Model file for the job. Use its own axes, mm. Face numbers are marked on the shaded views. A direction names the side the tool comes from. Coordinates: 2 decimals unless noted, no trailing zeros. Write each loop counter-clockwise with the first axis right and the second up, starting at its lowest first coordinate (ties: lowest second). Pieces come first, ordered by that corner, then holes.
Q1. Band-saw the part on B-B, the plane y = 74. Write the cut outline in (x, z), plus the area to 3 significant figures.
Q2. Pull direction X, two halves, no side cores. Call the marked faces 1, 2 and 3: released by +X, released by -X, zero draft, split by the parting line, or undercut.
Q3. Drill centre lines: probe 1 along X at (y, z) = (51.5, -21); probe 2 along Y at (x, z) = (24, -14); probe 3 along Z at (x, y) = (-20.75, 70.5). Where is each one in solid material? Low to high.
Q4. Pin check, flat tips, straight feed: P1, Ø5, axis at x = 22.5, y = 16.75, coming from the +Z side; P2, Ø9, axis at x = -22.5, y = 16.75, coming from the -Z side; P3, Ø1.3, axis at x = 25, y = 53, coming from the +Z side; P4, Ø3, axis at x = 15, z = -21, coming from the -Y side. Stop position of each tip, or through.
Q5. Band-saw the part on C-C, the plane z = -52. Write the cut outline in (x, y).
Q6. Band-saw the part on A-A, the plane x = 15.5. Write the cut outline in (y, z).
Q7. Band-saw the part on D-D, the plane x = 1. Write the cut outline in (y, z).
Q8. Which spindle directions (+Z, -Z, +X, -X, +Y, -Y) get a long thin tool onto all of the face, cutting with end or side? Do the marked faces 4 and 5. Say none if no direction does.
from build123d import *

# Parameters (mm, degrees)
SKETCH2_W           = 5
SKETCH2_H           = 50
BOSS_EXTRUDE1_DEPTH = 30
CUT_EXTRUDE1_REACH  = 66.607
SKETCH3_R           = 2.25
SKETCH6_W           = 47
SKETCH6_H           = 34
BOSS_EXTRUDE3_DEPTH = 60
SKETCH7_R           = 4
CUT_EXTRUDE2_DEPTH  = 2.3
CUT_EXTRUDE3_REACH  = 77.168
SKETCH8_R           = 11.5
SKETCH8_R_2         = 4.15
SKETCH8_R_3         = 1.75
CHAMFER1_SIZE       = 13
SKETCH9_R           = 3
CUT_EXTRUDE4_DEPTH  = 17
CHAMFER2_SIZE       = 9
SKETCH3_2_R         = 2.25
CUT_EXTRUDE5_DEPTH  = 5


with BuildPart() as part:
    # Sketch2 → Boss-Extrude1 (new, symmetric)
    with BuildSketch(Plane(origin=(0, 0, 0), x_dir=(0, 0, -1), z_dir=(1, 0, 0))):
        with Locations((13, 32)):
            Rectangle(SKETCH2_W, SKETCH2_H)
    extrude(amount=BOSS_EXTRUDE1_DEPTH, both=True)

    # Sketch3 → Cut-Extrude1 (cut, up to next)
    with BuildSketch(Plane.XY.offset(-10.5), mode=Mode.PRIVATE) as cut_extrude1_sk1:
        with Locations((-22.5, 16.75)):
            Circle(SKETCH3_R)
    cut_extrude1_tool1 = extrude(cut_extrude1_sk1.sketch, amount=-CUT_EXTRUDE1_REACH, mode=Mode.PRIVATE) & part.part
    # Sketch3 → Cut-Extrude1 (cut, up to next)
    with BuildSketch(Plane.XY.offset(-10.5), mode=Mode.PRIVATE) as cut_extrude1_sk2:
        with Locations((-7.5, 16.75)):
            Circle(SKETCH3_R)
    cut_extrude1_tool2 = extrude(cut_extrude1_sk2.sketch, amount=-CUT_EXTRUDE1_REACH, mode=Mode.PRIVATE) & part.part
    # Sketch3 → Cut-Extrude1 (cut, up to next)
    with BuildSketch(Plane.XY.offset(-10.5), mode=Mode.PRIVATE) as cut_extrude1_sk3:
        with Locations((7.5, 16.75)):
            Circle(SKETCH3_R)
    cut_extrude1_tool3 = extrude(cut_extrude1_sk3.sketch, amount=-CUT_EXTRUDE1_REACH, mode=Mode.PRIVATE) & part.part
    # Sketch3 → Cut-Extrude1 (cut, up to next)
    with BuildSketch(Plane.XY.offset(-10.5), mode=Mode.PRIVATE) as cut_extrude1_sk4:
        with Locations((22.5, 16.75)):
            Circle(SKETCH3_R)
    cut_extrude1_tool4 = extrude(cut_extrude1_sk4.sketch, amount=-CUT_EXTRUDE1_REACH, mode=Mode.PRIVATE) & part.part
    # Sketch3 → Cut-Extrude1 (cut, up to next)
    with BuildSketch(Plane.XY.offset(-10.5), mode=Mode.PRIVATE) as cut_extrude1_sk5:
        with Locations((-24, 52)):
            Circle(SKETCH3_R)
    cut_extrude1_tool5 = extrude(cut_extrude1_sk5.sketch, amount=-CUT_EXTRUDE1_REACH, mode=Mode.PRIVATE) & part.part
    # Sketch3 → Cut-Extrude1 (cut, up to next)
    with BuildSketch(Plane.XY.offset(-10.5), mode=Mode.PRIVATE) as cut_extrude1_sk6:
        with Locations((-6, 52)):
            Circle(SKETCH3_R)
    cut_extrude1_tool6 = extrude(cut_extrude1_sk6.sketch, amount=-CUT_EXTRUDE1_REACH, mode=Mode.PRIVATE) & part.part
    # Sketch3 → Cut-Extrude1 (cut, up to next)
    with BuildSketch(Plane.XY.offset(-10.5), mode=Mode.PRIVATE) as cut_extrude1_sk7:
        with Locations((-24, 28)):
            Circle(SKETCH3_R)
    cut_extrude1_tool7 = extrude(cut_extrude1_sk7.sketch, amount=-CUT_EXTRUDE1_REACH, mode=Mode.PRIVATE) & part.part
    # Sketch3 → Cut-Extrude1 (cut, up to next)
    with BuildSketch(Plane.XY.offset(-10.5), mode=Mode.PRIVATE) as cut_extrude1_sk8:
        with Locations((-6, 28)):
            Circle(SKETCH3_R)
    cut_extrude1_tool8 = extrude(cut_extrude1_sk8.sketch, amount=-CUT_EXTRUDE1_REACH, mode=Mode.PRIVATE) & part.part
    # Sketch3 → Cut-Extrude1 (cut, up to next)
    with BuildSketch(Plane.XY.offset(-10.5), mode=Mode.PRIVATE) as cut_extrude1_sk9:
        with Locations(Location((6, 28, 0), (0, 0, 90))):
            Circle(SKETCH3_R)
    cut_extrude1_tool9 = extrude(cut_extrude1_sk9.sketch, amount=-CUT_EXTRUDE1_REACH, mode=Mode.PRIVATE) & part.part
    # Sketch3 → Cut-Extrude1 (cut, up to next)
    with BuildSketch(Plane.XY.offset(-10.5), mode=Mode.PRIVATE) as cut_extrude1_sk10:
        with Locations(Location((24, 28, 0), (0, 0, 90))):
            Circle(SKETCH3_R)
    cut_extrude1_tool10 = extrude(cut_extrude1_sk10.sketch, amount=-CUT_EXTRUDE1_REACH, mode=Mode.PRIVATE) & part.part
    # Sketch3 → Cut-Extrude1 (cut, up to next)
    with BuildSketch(Plane.XY.offset(-10.5), mode=Mode.PRIVATE) as cut_extrude1_sk11:
        with Locations(Location((6, 52, 0), (0, 0, 90))):
            Circle(SKETCH3_R)
    cut_extrude1_tool11 = extrude(cut_extrude1_sk11.sketch, amount=-CUT_EXTRUDE1_REACH, mode=Mode.PRIVATE) & part.part
    # Sketch3 → Cut-Extrude1 (cut, up to next)
    with BuildSketch(Plane.XY.offset(-10.5), mode=Mode.PRIVATE) as cut_extrude1_sk12:
        with Locations(Location((24, 52, 0), (0, 0, 90))):
            Circle(SKETCH3_R)
    cut_extrude1_tool12 = extrude(cut_extrude1_sk12.sketch, amount=-CUT_EXTRUDE1_REACH, mode=Mode.PRIVATE) & part.part
    add(cut_extrude1_tool1.solids().sort_by_distance((-22.5, 16.75, -10.5))[0], mode=Mode.SUBTRACT)
    add(cut_extrude1_tool2.solids().sort_by_distance((-7.5, 16.75, -10.5))[0], mode=Mode.SUBTRACT)
    add(cut_extrude1_tool3.solids().sort_by_distance((7.5, 16.75, -10.5))[0], mode=Mode.SUBTRACT)
    add(cut_extrude1_tool4.solids().sort_by_distance((22.5, 16.75, -10.5))[0], mode=Mode.SUBTRACT)
    add(cut_extrude1_tool5.solids().sort_by_distance((-24, 52, -10.5))[0], mode=Mode.SUBTRACT)
    add(cut_extrude1_tool6.solids().sort_by_distance((-6, 52, -10.5))[0], mode=Mode.SUBTRACT)
    add(cut_extrude1_tool7.solids().sort_by_distance((-24, 28, -10.5))[0], mode=Mode.SUBTRACT)
    add(cut_extrude1_tool8.solids().sort_by_distance((-6, 28, -10.5))[0], mode=Mode.SUBTRACT)
    add(cut_extrude1_tool9.solids().sort_by_distance((6, 28, -10.5))[0], mode=Mode.SUBTRACT)
    add(cut_extrude1_tool10.solids().sort_by_distance((24, 28, -10.5))[0], mode=Mode.SUBTRACT)
    add(cut_extrude1_tool11.solids().sort_by_distance((6, 52, -10.5))[0], mode=Mode.SUBTRACT)
    add(cut_extrude1_tool12.solids().sort_by_distance((24, 52, -10.5))[0], mode=Mode.SUBTRACT)

    # Sketch6 → Boss-Extrude3 (add)
    with BuildSketch(Plane(origin=(30, 0, 0), x_dir=(0, 0, -1), z_dir=(1, 0, 0))):
        with Locations((34, 62)):
            Rectangle(SKETCH6_W, SKETCH6_H)
    extrude(amount=-BOSS_EXTRUDE3_DEPTH)

    # Sketch7 → Cut-Extrude2 (cut)
    with BuildSketch(Plane(origin=(0, 0, -15.5), x_dir=(-1, 0, 0), z_dir=(0, 0, -1))):
        with Locations(Location((22.5, 16.75, 0), (0, 0, 90))):
            Circle(SKETCH7_R)
        with Locations(Location((24, 28, 0), (0, 0, 90))):
            Circle(SKETCH7_R)
        with Locations(Location((7.5, 16.75, 0), (0, 0, 90))):
            Circle(SKETCH7_R)
        with Locations(Location((-7.5, 16.75, 0), (0, 0, 90))):
            Circle(SKETCH7_R)
        with Locations(Location((-22.5, 16.75, 0), (0, 0, 90))):
            Circle(SKETCH7_R)
        with Locations(Location((6, 28, 0), (0, 0, 90))):
            Circle(SKETCH7_R)
        with Locations(Location((-6, 28, 0), (0, 0, 270))):
            Circle(SKETCH7_R)
        with Locations(Location((-24, 28, 0), (0, 0, 270))):
            Circle(SKETCH7_R)
    extrude(amount=-CUT_EXTRUDE2_DEPTH, mode=Mode.SUBTRACT)

    # Sketch8 → Cut-Extrude3 (cut, up to next)
    with BuildSketch(Plane.XZ.offset(-45), mode=Mode.PRIVATE) as cut_extrude3_sk1:
        with Locations(Location((0, -36.5, 0), (0, 0, 270))):
            Circle(SKETCH8_R)
    cut_extrude3_tool1 = extrude(cut_extrude3_sk1.sketch, amount=-CUT_EXTRUDE3_REACH, mode=Mode.PRIVATE) & part.part
    # Sketch8 → Cut-Extrude3 (cut, up to next)
    with BuildSketch(Plane.XZ.offset(-45), mode=Mode.PRIVATE) as cut_extrude3_sk2:
        with Locations(Location((-20.75, -36.5, 0), (0, 0, 270))):
            Circle(SKETCH8_R_2)
    cut_extrude3_tool2 = extrude(cut_extrude3_sk2.sketch, amount=-CUT_EXTRUDE3_REACH, mode=Mode.PRIVATE) & part.part
    # Sketch8 → Cut-Extrude3 (cut, up to next)
    with BuildSketch(Plane.XZ.offset(-45), mode=Mode.PRIVATE) as cut_extrude3_sk3:
        with Locations(Location((20.75, -36.5, 0), (0, 0, 90))):
            Circle(SKETCH8_R_2)
    cut_extrude3_tool3 = extrude(cut_extrude3_sk3.sketch, amount=-CUT_EXTRUDE3_REACH, mode=Mode.PRIVATE) & part.part
    # Sketch8 → Cut-Extrude3 (cut, up to next)
    with BuildSketch(Plane.XZ.offset(-45), mode=Mode.PRIVATE) as cut_extrude3_sk4:
        with Locations(Location((-15.5, -52, 0), (0, 0, 270))):
            Circle(SKETCH8_R_3)
    cut_extrude3_tool4 = extrude(cut_extrude3_sk4.sketch, amount=-CUT_EXTRUDE3_REACH, mode=Mode.PRIVATE) & part.part
    # Sketch8 → Cut-Extrude3 (cut, up to next)
    with BuildSketch(Plane.XZ.offset(-45), mode=Mode.PRIVATE) as cut_extrude3_sk5:
        with Locations(Location((15.5, -52, 0), (0, 0, 90))):
            Circle(SKETCH8_R_3)
    cut_extrude3_tool5 = extrude(cut_extrude3_sk5.sketch, amount=-CUT_EXTRUDE3_REACH, mode=Mode.PRIVATE) & part.part
    # Sketch8 → Cut-Extrude3 (cut, up to next)
    with BuildSketch(Plane.XZ.offset(-45), mode=Mode.PRIVATE) as cut_extrude3_sk6:
        with Locations(Location((15.5, -21, 0), (0, 0, 270))):
            Circle(SKETCH8_R_3)
    cut_extrude3_tool6 = extrude(cut_extrude3_sk6.sketch, amount=-CUT_EXTRUDE3_REACH, mode=Mode.PRIVATE) & part.part
    # Sketch8 → Cut-Extrude3 (cut, up to next)
    with BuildSketch(Plane.XZ.offset(-45), mode=Mode.PRIVATE) as cut_extrude3_sk7:
        with Locations(Location((-15.5, -21, 0), (0, 0, 90))):
            Circle(SKETCH8_R_3)
    cut_extrude3_tool7 = extrude(cut_extrude3_sk7.sketch, amount=-CUT_EXTRUDE3_REACH, mode=Mode.PRIVATE) & part.part
    add(cut_extrude3_tool1.solids().sort_by_distance((0, 45, -36.5))[0], mode=Mode.SUBTRACT)
    add(cut_extrude3_tool2.solids().sort_by_distance((-20.75, 45, -36.5))[0], mode=Mode.SUBTRACT)
    add(cut_extrude3_tool3.solids().sort_by_distance((20.75, 45, -36.5))[0], mode=Mode.SUBTRACT)
    add(cut_extrude3_tool4.solids().sort_by_distance((-15.5, 45, -52))[0], mode=Mode.SUBTRACT)
    add(cut_extrude3_tool5.solids().sort_by_distance((15.5, 45, -52))[0], mode=Mode.SUBTRACT)
    add(cut_extrude3_tool6.solids().sort_by_distance((15.5, 45, -21))[0], mode=Mode.SUBTRACT)
    add(cut_extrude3_tool7.solids().sort_by_distance((-15.5, 45, -21))[0], mode=Mode.SUBTRACT)

    # Chamfer1
    chamfer1_edges = [part.edges().sort_by_distance(p)[0] for p in [
        (30, 62, -57.5),
        (-30, 62, -57.5),
    ]]
    chamfer(chamfer1_edges, length=CHAMFER1_SIZE)

    # Sketch9 → Cut-Extrude4 (cut)
    with BuildSketch(Plane.XZ.offset(-45)):
        with Locations(Location((-15.5, -21, 0), (0, 0, 270))):
            Circle(SKETCH9_R)
        with Locations(Location((-15.5, -52, 0), (0, 0, 270))):
            Circle(SKETCH9_R)
        with Locations(Location((15.5, -52, 0), (0, 0, 90))):
            Circle(SKETCH9_R)
        with Locations(Location((15.5, -21, 0), (0, 0, 90))):
            Circle(SKETCH9_R)
    extrude(amount=-CUT_EXTRUDE4_DEPTH, mode=Mode.SUBTRACT)

    # Chamfer2
    # the kernel refuses this chamfer: 9 mm, written as the material it takes off along each edge
    with BuildSketch(Plane(origin=(30, 79, -67.645146892), x_dir=(-0.9996219169112966, 0.027495876610586775, 0), z_dir=(0, 0, 1)), Plane(origin=(-30, 79, -67.645146892), x_dir=(-0.027495876610586386, -0.9996219169112969, 0), z_dir=(0, 0, 1))) as chamfer2_piece_1:
        Polygon((CHAMFER2_SIZE * 0.999621916911, CHAMFER2_SIZE * 0.0274958766106), (-CHAMFER2_SIZE * 0.0274958766106, CHAMFER2_SIZE * 0.999621916911), (0, 0), align=None)
    extrude(amount=80.290293783, mode=Mode.SUBTRACT)

    # Sketch3<2> → Cut-Extrude5 (cut)
    with BuildSketch(Plane.XY.offset(-10.5)):
        with Locations((-22.5, 16.75)):
            Circle(SKETCH3_2_R)
        with Locations((-7.5, 16.75)):
            Circle(SKETCH3_2_R)
        with Locations((7.5, 16.75)):
            Circle(SKETCH3_2_R)
        with Locations((22.5, 16.75)):
            Circle(SKETCH3_2_R)
        with Locations((-24, 52)):
            Circle(SKETCH3_2_R)
        with Locations((-6, 52)):
            Circle(SKETCH3_2_R)
        with Locations((-24, 28)):
            Circle(SKETCH3_2_R)
        with Locations((-6, 28)):
            Circle(SKETCH3_2_R)
        with Locations(Location((6, 28, 0), (0, 0, 270))):
            Circle(SKETCH3_2_R)
        with Locations(Location((24, 28, 0), (0, 0, 270))):
            Circle(SKETCH3_2_R)
        with Locations(Location((6, 52, 0), (0, 0, 90))):
            Circle(SKETCH3_2_R)
        with Locations(Location((24, 52, 0), (0, 0, 90))):
            Circle(SKETCH3_2_R)
    extrude(amount=-CUT_EXTRUDE5_DEPTH, mode=Mode.SUBTRACT)


solid = part.part
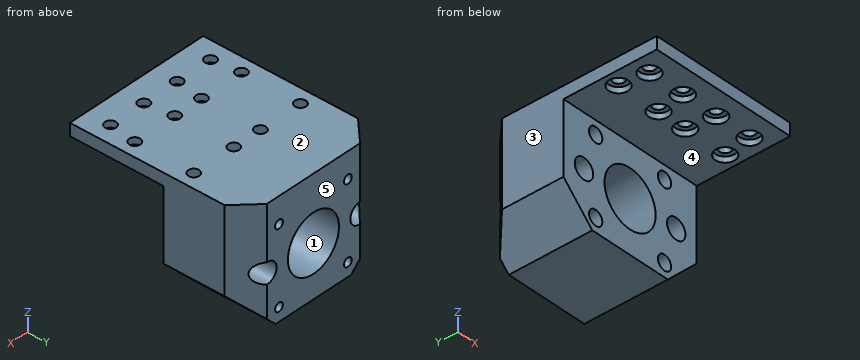
Answer sheet:
1. outline: (-26, -48.5) - (-17, -57.5) - (17, -57.5) - (26, -48.5) - (26, -10.5) - (-26, -10.5) - close; hole circle Ø8.3 at (-20.75, -36.5); hole circle Ø3.5 at (-15.5, -52); hole circle Ø3.5 at (-15.5, -21); hole circle Ø23 at (0, -36.5); hole circle Ø3.5 at (15.5, -52); hole circle Ø3.5 at (15.5, -21); hole circle Ø8.3 at (20.75, -36.5)
1. area: 1,800 mm2
2. face 1: undercut
2. face 2: zero draft
2. face 3: released by -X
3. probe 1: x = -30 to -18.5, -12.5 to 12.5, 18.5 to 30
3. probe 2: y = 7 to 13.04, 20.46 to 24, 32 to 49.75, 54.25 to 76
3. probe 3: z = -53.75 to -40.65, -32.35 to -10.5
4. P1: stops at z = -10.5
4. P2: stops at z = -15.5
4. P3: stops at z = -15.5
4. P4: stops at y = 62
5. outline: (-22.5, 45) - (-18.5, 45) - (-18.5, 62) - (-17.25, 62) - (-17.25, 79) - (-21, 79) - (-22.5, 77.5) - close; (-13.75, 62) - (-12.5, 62) - (-12.5, 45) - (12.5, 45) - (12.5, 62) - (13.75, 62) - (13.75, 79) - (-13.75, 79) - close; (17.25, 62) - (18.5, 62) - (18.5, 45) - (22.5, 45) - (22.5, 77.5) - (21, 79) - (17.25, 79) - close
6. outline: (7, -15.5) - (45, -15.5) - (45, -18) - (62, -18) - (62, -19.25) - (79, -19.25) - (79, -10.5) - (7, -10.5) - close; (45, -57.5) - (79, -57.5) - (79, -53.75) - (62, -53.75) - (62, -55) - (45, -55) - close; (45, -49) - (62, -49) - (62, -50.25) - (79, -50.25) - (79, -22.75) - (62, -22.75) - (62, -24) - (45, -24) - close
7. outline: (7, -15.5) - (45, -15.5) - (45, -25.04) - (79, -25.04) - (79, -10.5) - (7, -10.5) - close; (45, -57.5) - (79, -57.5) - (79, -47.96) - (45, -47.96) - close
8. face 4: -Z, +X, -X, -Y
8. face 5: +Z, -Z, +X, -X, +Y
